Can you work these out from the drawing? Everything is in mm from the part's minimum corner. Coordinates: 2 decimals unless noted, no trailing zeros. Loops run counter-clockwise (first coordinate to the right, second up) from the corner with the lowest first, then second, coordinate; pieces in that order, holes last.
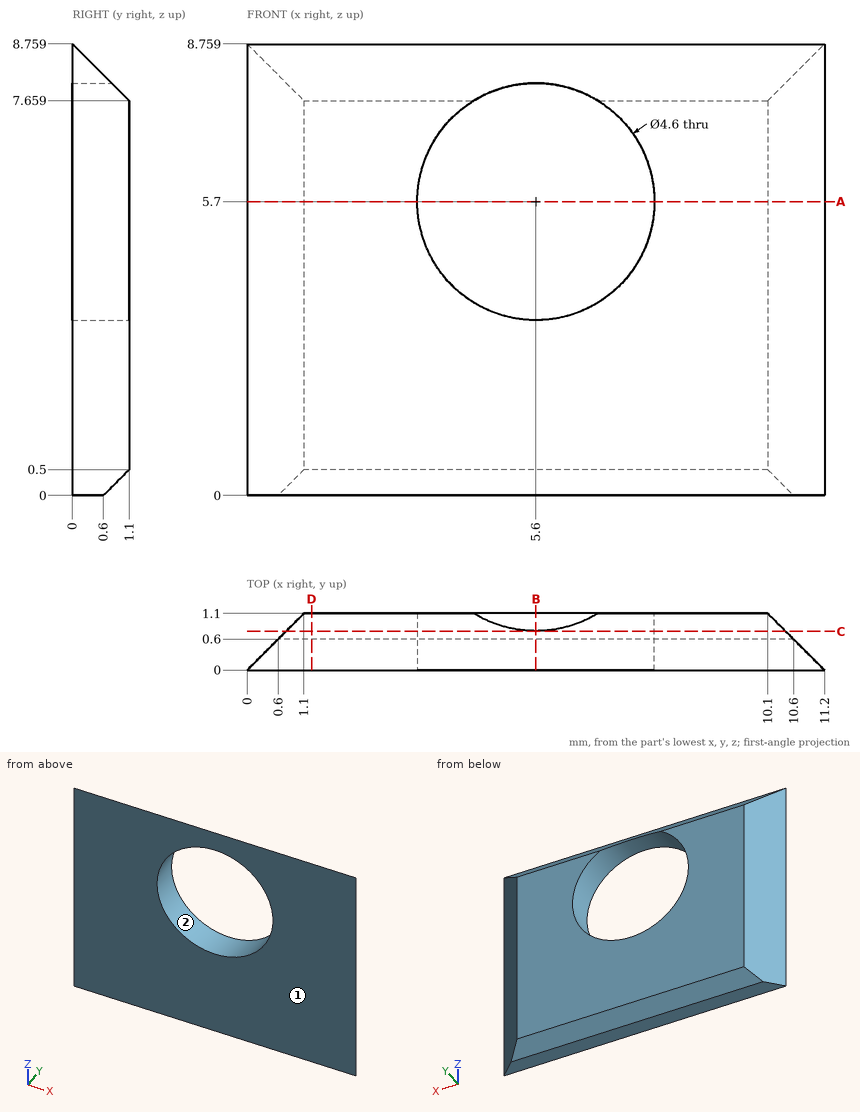
1. We'd pull the mould along Z, two halves only. Please class the marked faces 1 and 2: +Z half, -Z half, draft (parallel to the pull), parting line (faces both ways), or undercut.
2. I want a section at B-B (x = 5.6). Please give me the cut outline in (y, z).
3. I want a section at D-D (x = 1.25). Please give me the cut outline in (y, z).
4. I need wall thicknesses on line 1 along Z through (x, y) = (7.5, 0.55) (1 decimal); line 2 along Z through (x, y) = (4.75, 0.2) (1 decimal); line 3 along X through (y, z) = (0.25, 7.25). Which ranges of each line are inside material? Lowest first, please.
5. I want a section at A-A (z = 5.7). Please give me the cut outline in (x, y).
6. I want a section at C-C (y = 0.75). Please give me the cut outline in (x, z).
7. For pin 1 (3 mm diameter, centred on x = 5.6, z = 5.7, fed in from -Y), with a flat end and sliding along its axis, tell me the tip position at first contact or that it passes through.
Response values:
1. face 1: draft
1. face 2: undercut
2. outline: (0, 0) - (0.6, 0) - (1.1, 0.5) - (1.1, 3.4) - (0, 3.4) - close; (0, 8) - (0.76, 8) - (0, 8.76) - close
3. outline: (0, 0) - (0.6, 0) - (1.1, 0.5) - (1.1, 7.66) - (0, 8.76) - close
4. line 1: z = 0 to 4.4, 7 to 8.2
4. line 2: z = 0 to 3.6, 7.8 to 8.6
4. line 3: x = 0.25 to 3.9, 7.3 to 10.95
5. outline: (0, 0) - (3.3, 0) - (3.3, 1.1) - (1.1, 1.1) - close; (7.9, 0) - (11.2, 0) - (10.1, 1.1) - (7.9, 1.1) - close
6. outline: (0.75, 0.15) - (10.45, 0.15) - (10.45, 8.01) - (0.75, 8.01) - close; hole circle Ø4.6 at (5.6, 5.7)
7. pin 1: passes through
